```python
from build123d import *
from OCP.BRepFilletAPI import BRepFilletAPI_MakeChamfer

# Parameters (mm, degrees)
BOSS_EXTRUDE1_DEPTH = 5
SKETCH4_R           = 2
CUT_EXTRUDE2_DEPTH  = 10
CHAMFER1_SIZE       = 0.5
CHAMFER1_SIZE2      = 0.181985117


with BuildPart() as part:
    # Sketch2 → Boss-Extrude1 (new body)
    with BuildSketch(Plane.YZ):
        Polygon((-3, 8), (-13, 8), (-13, 3), (-3, 3), (2, 3), (5, 0), (13.351646544, 5.5), (5, 11), (2, 8), align=None)
    extrude(amount=BOSS_EXTRUDE1_DEPTH)

    # Sketch4 → Cut-Extrude2 (cut)
    with BuildSketch(Plane.XY.offset(8)):
        with Locations((2.5, -8)):
            Circle(SKETCH4_R)
    extrude(amount=-CUT_EXTRUDE2_DEPTH, mode=Mode.SUBTRACT)

    # Chamfer1: one chamfer whose edges measure the first distance from different faces: ONE call of the kernel's chamfer builder (chamfer() names one face for all edges)
    chamfer1_edges_1 = [part.edges().sort_by_distance(p)[0] for p in [
        (0, -13, 5.5),
    ]]
    chamfer1_side_1 = [part.faces().sort_by_distance(p)[0] for p in [
        (0, 0.23145202, 5.5),
    ]]
    chamfer1_edges_2 = [part.edges().sort_by_distance(p)[0] for p in [
        (2.5, -13, 3),
    ]]
    chamfer1_side_2 = [part.faces().sort_by_distance(p)[0] for p in [
        (2.5, -4.996810824, 3),
    ]]
    chamfer1_edges_3 = [part.edges().sort_by_distance(p)[0] for p in [
        (2.5, -13, 8),
    ]]
    chamfer1_side_3 = [part.faces().sort_by_distance(p)[0] for p in [
        (2.5, -4.996810824, 8),
    ]]
    chamfer1_edges_4 = [part.edges().sort_by_distance(p)[0] for p in [
        (5, -13, 5.5),
    ]]
    chamfer1_side_4 = [part.faces().sort_by_distance(p)[0] for p in [
        (5, 0.23145202, 5.5),
    ]]
    chamfer1 = BRepFilletAPI_MakeChamfer(part.part.solid().wrapped)
    for e in chamfer1_edges_1:
        chamfer1.Add(CHAMFER1_SIZE, CHAMFER1_SIZE2, e.wrapped, chamfer1_side_1[0].wrapped)  # the first distance lies on this face
    for e in chamfer1_edges_2:
        chamfer1.Add(CHAMFER1_SIZE, CHAMFER1_SIZE2, e.wrapped, chamfer1_side_2[0].wrapped)  # the first distance lies on this face
    for e in chamfer1_edges_3:
        chamfer1.Add(CHAMFER1_SIZE, CHAMFER1_SIZE2, e.wrapped, chamfer1_side_3[0].wrapped)  # the first distance lies on this face
    for e in chamfer1_edges_4:
        chamfer1.Add(CHAMFER1_SIZE, CHAMFER1_SIZE2, e.wrapped, chamfer1_side_4[0].wrapped)  # the first distance lies on this face
    add(Compound.cast(chamfer1.Shape()), mode=Mode.REPLACE)


solid = part.part
```
For this review, take the finished solid that the model builds, in its own axes (mm). A direction names the side the tool comes from. Coordinates: 2 decimals unless noted, no trailing zeros. Order: outer loops, then holes, each group sorted by start corner. A loop starts at its lowest first (then second) coordinate and runs counter-clockwise, first axis right, second up. Notation, with made-up numbers: (40.25, 17) - (53.25, 17) arc R13 cw to (53.25, 25) - close; hole circle Ø1 at (41.5, -20.75). An arc over 180 degrees is marked (long way). Answer as a JSON object with one key per item and string values. Group by question number.
1. We need section D-D on y = -0.75. State the section outline as (x, z) points.
2. For probe 1 along Z at (x, y) = (3.95, -2); probe 2 along Y at (x, z) = (4.25, 6.25); probe 3 along X at (y, z) = (-9.5, 5.25), list the stretches that pass through material, from the lowest coordinate up.
3. The part is to be moulded in two halves that separate along Y. For faces 4 (the flat face through (2.465, 9.234, 8.212)), 5 (the flat face through (2, 3, 2)), 6 (the cylindrical face through (2.24, -6.017, 5.535)), say which applies: pulls with the +Y half, pulls with the -Y half, needs draft (parallel to the pull), parting line crosses it, or undercut.
4. We need section B-B on x = 2.4. State the section outline as (y, z) points, then the cut area to 3 significant figures.
5. For faces 1 (the flat face through (2, -5, 8)), 2 (the flat face through (2, -5, 3)), 3 (the flat face through (0, 0, 6)), list the 3-axis set-ups (+Z, -Z, +X, -X, +Y, -Y) from which the entire face can be reached by the end or side of a thin tool; tool diameter is ignored.
6. We need section A-A on y = -8. State the section outline as (x, z) points.
7. Clearance check with flat-ended pins moving along their axes: P1, Ø2, axis at x = 1, y = 7.5, coming from the -Z side; P2, Ø2, axis at x = 1.5, y = -3, coming from the +Z side. State where each tip first meets the part, or that it passes through.
8. We need section C-C on z = 8.75. State the section outline as (x, y) points, then the cut area to 3 significant figures.
Final values:
{
 "1": {"outline": "(0, 3) - (5, 3) - (5, 8) - (0, 8) - close"},
 "2": {"probe 1": "3 to 8", "probe 2": "-13 to -8.97, -7.03 to 12.21", "probe 3": "0 to 1.18, 3.82 to 5"},
 "3": {"face 4": "pulls with the +Y half", "face 5": "pulls with the -Y half", "face 6": "undercut"},
 "4": {"outline": "(-13, 3.18) - (-12.5, 3) - (-10, 3) - (-10, 8) - (-12.5, 8) - (-13, 7.82) - close; (-6, 3) - (2, 3) - (5, 0) - (13.35, 5.5) - (5, 11) - (2, 8) - (-6, 8) - close", "area": "125 mm²"},
 "5": {"face 1": "+Z, +X, -X, -Y", "face 2": "-Z, +X, -X, -Y", "face 3": "+Z, -Z, -X, +Y, -Y"},
 "6": {"outline": "(0, 3) - (0.5, 3) - (0.5, 8) - (0, 8) - close; (4.5, 3) - (5, 3) - (5, 8) - (4.5, 8) - close"},
 "7": {"P1": "z = 0.99", "P2": "z = 8"},
 "8": {"outline": "(0, 2.75) - (5, 2.75) - (5, 8.42) - (0, 8.42) - close", "area": "28.3 mm²"}
}
